Source: CAD feature listing. Evaluate the final solid. Frame: model axes, mm. Face numbers are marked on the shaded views. A direction names the side the tool comes from. Give positions to 0.01 mm unless a question says otherwise; leave off trailing zeros. Write each loop counter-clockwise with the first axis right and the second up, starting at its lowest first coordinate (ties: lowest second). Pieces come first, ordered by that corner, then holes. Notation, with made-up numbers: (-12, 28) -> (0, 28) arc R26 cw to (0, 55) -> close; hole circle Ø11 at (60, 81). An arc over 180 degrees is marked (long way). Write item = value, one per line.
Solid Edge part; units mm, degrees
sketch "Sketch1" plane through (0, 0, 0) normal (0, -1, 0) x (1, 0, 0)
  line L0 (37.5, 26) -> (-37.5, 26)
  line L1 (-37.5, 26) -> (-37.5, -26)
  line L2 (-37.5, -26) -> (37.5, -26)
  line L3 (37.5, -26) -> (37.5, 26)
extrude "Protrusion1" add sketch "Sketch1" against normal blind 15
sketch "Sketch2" plane through (0, 0, 0) normal (0, -1, 0) x (1, 0, 0)
  circle A0 centre (-27.5, 16) radius 5
  circle A1 centre (27.5, 16) radius 5
  circle A2 centre (27.5, -16) radius 5
  circle A3 centre (-27.5, -16) radius 5
extrude "Cutout1" cut sketch "Sketch2" against normal up to next
sketch "Sketch3" plane through (0, 0, 0) normal (0, -1, 0) x (1, 0, 0)
  line L0 (-32.5, 6) -> (-12.5, 6)
  line L1 (-12.5, 6) -> (-12.5, -6)
  line L2 (-12.5, -6) -> (-32.5, -6)
  line L3 (-32.5, -6) -> (-32.5, 6)
extrude "ExtrudedProtrusion_3" add sketch "Sketch3" along normal blind 10
sketch "Sketch4" plane through (-22.5, -10, 0) normal (0, -1, 0) x (1, 0, 0)
  line L0 (-10, 6) -> (10, 6)
  line L1 (10, 6) -> (10, -6)
  line L2 (10, -6) -> (-10, -6)
  line L3 (-10, -6) -> (-10, 6)
revolve "RevolvedProtrusion_2" add sketch "Sketch4" angle 90 about axis through (-2.5, -10, -6) along (0, 0, 1)
sketch "Sketch5" plane through (-2.5, -30, 0) normal (1, 0, 0) x (0, 0, 1)
  line L0 (-6, 10) -> (6, 10)
  line L1 (6, 10) -> (6, -10)
  line L2 (6, -10) -> (-6, -10)
  line L3 (-6, -10) -> (-6, 10)
extrude "ExtrudedProtrusion_4" add sketch "Sketch5" along normal blind 10
sketch "Sketch6" plane through (-12.5, -20, 0) normal (0, 0, -1) x (0, -1, 0)
  line L0 (20, -28) -> (20, -19)
  line L1 (20, -19) -> (0, -19)
  line L2 (0, -19) -> (0, -20)
  line L3 (0, -20) -> (0, -28)
  line L4 (0, -28) -> (20, -28)
revolve "RevolvedProtrusion1" add sketch "Sketch6" angle 360 about axis through (23.5, -40, 0) along (0, 1, 0)
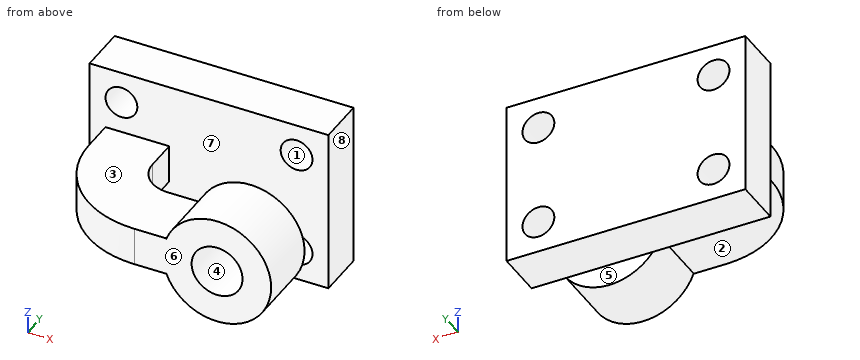
1) Access query for the marked faces 1, 2, 3 and 4. Directions: +Z, -Z, +X, -X, +Y, -Y. A direction counts if a zero-diameter tool reaches every point of the face in a straight line with its end or side. Return the directions, or none.
Computed:
face_1 = +Y
face_2 = -Z, -X, -Y
face_3 = +Z, -X, -Y
face_4 = -Y
2) Contact query for flat-ended pins moving along their axis: pin 1 (5 mm diameter, centred on y = 0.5, z = -10, fed in from +X); pin 2 (16 mm diameter, centred on x = -27.5, z = -16, fed in from -Y); pin 3 (6 mm diameter, centred on y = -15, z = 7, fed in from -X). Output: stop coordinate, or through.
Computed:
pin_1 = 37.5
pin_2 = 0
pin_3 = -32.42
3) Cut plane C-C (x = 2.5). Return the cut outline in (y, z).
Computed:
outline = (-40, -6) -> (-20, -6) -> (-20, 6) -> (-40, 6) -> close; (0, -26) -> (15, -26) -> (15, 26) -> (0, 26) -> close
4) Cut plane A-A (x = 23.5). Return the cut outline in (y, z).
Computed:
outline = (-40, -17) -> (-20, -17) -> (-20, -8) -> (-40, -8) -> close; (-40, 8) -> (-20, 8) -> (-20, 17) -> (-40, 17) -> close; (0, -26) -> (15, -26) -> (15, -19) -> (0, -19) -> close; (0, -13) -> (15, -13) -> (15, 13) -> (0, 13) -> close; (0, 19) -> (15, 19) -> (15, 26) -> (0, 26) -> close
5) Cut plane B-B (z = 20). Return the cut outline in (x, y).
Computed:
outline = (-37.5, 0) -> (-30.5, 0) -> (-30.5, 15) -> (-37.5, 15) -> close; (-24.5, 0) -> (24.5, 0) -> (24.5, 15) -> (-24.5, 15) -> close; (30.5, 0) -> (37.5, 0) -> (37.5, 15) -> (30.5, 15) -> close
6) Cut plane D-D (y = -26). Return the cut outline in (x, z), then the cut area to 3 significant figures.
Computed:
outline = (-27.88, -6) -> (7.5, -6) -> (7.5, -5.74) arc R17 ccw (long way) to (7.5, 5.74) -> (7.5, 6) -> (-27.88, 6) -> close; hole circle Ø16 at (23.5, 0)
area = 1,120 mm²
7) Material intervals for L1, parallel to Z at x = 27.5, y = 11.5; L2, parallel to Y at x = 15, z = 10; L3, parallel to X at y = 1, z = -14, sorted ascending.
Computed:
L1 = -26 to -21, -11 to 11, 21 to 26
L2 = -40 to -20, 0 to 15
L3 = -37.5 to -32.08, -22.92 to 22.92, 32.08 to 37.5
8) Draft query along Y for the marked faces 5, 6, 7 and 8. Return one class per face: pulls with the +Y half, pulls with the -Y half, needs draft (parallel to the pull), parting line crosses it, or undercut.
Computed:
face_5 = undercut
face_6 = pulls with the -Y half
face_7 = undercut
face_8 = needs draft
